from build123d import *

# Parameters (mm, degrees)
SKETCH_W        = 90
SKETCH_H        = 130
PAD_DEPTH       = 3
PAD007_DEPTH    = 3
PAD006_DEPTH    = 3
SKETCH014_R     = 5
SKETCH014_R_2   = 2
POCKET004_DEPTH = 10
SKETCH015_W     = 131.132767
SKETCH015_H     = 1
POCKET005_DEPTH = 100


with BuildPart() as pad007:
    # Sketch → Pad (new body)
    with BuildSketch(Plane.XY):
        with Locations((45, 65)):
            Rectangle(SKETCH_W, SKETCH_H)
    extrude(amount=PAD_DEPTH)

    # Sketch006 → Pad007 (new body)
    with BuildSketch(Plane.XY.offset(3)):
        with BuildLine():
            Line((0, 0), (90, 0))
            Line((90, 0), (90, 31.200001))
            Line((90, 87.7297593266), (90, 31.200001))
            Line((63.384261619, 87.7297593266), (90, 87.7297593266))
            ThreePointArc((73.2419105019, 65.6401585516), (70.414665309, 77.6228043326), (63.384261619, 87.7297593266))
            ThreePointArc((61.470024, 41.9983394519), (70.1525128312, 52.4267750542), (73.2419105019, 65.6401585516))
            Line((61.470024, 31.2), (61.470024, 41.9983394519))
            Line((0, 31.2), (61.470024, 31.2))
            Line((0, 31.2), (0, 0))
        make_face()
    extrude(amount=PAD007_DEPTH)


with BuildPart() as pocket005:
    # Sketch008 → Pad006 (new body)
    with BuildSketch(Plane(origin=(90, 130, 3), x_dir=(-1, 0, 0), z_dir=(0, 0, 1))):
        with BuildLine():
            Line((0, 0), (90, 0))
            Line((90, 0), (90, 31.200001))
            Line((90, 87.7297593266), (90, 31.200001))
            Line((63.384261619, 87.7297593266), (90, 87.7297593266))
            ThreePointArc((73.2419105019, 65.6401585516), (70.414665309, 77.6228043326), (63.384261619, 87.7297593266))
            ThreePointArc((61.470024, 41.9983394519), (70.1525128312, 52.4267750542), (73.2419105019, 65.6401585516))
            Line((61.470024, 31.2), (61.470024, 41.9983394519))
            Line((0, 31.2), (61.470024, 31.2))
            Line((0, 31.2), (0, 0))
        make_face()
    extrude(amount=PAD006_DEPTH)

    # Fusion: union Pad007
    add(pad007.part)

    # Sketch014 → Pocket004 (cut)
    with BuildSketch(Plane(origin=(0, 0, 0), x_dir=(1, 0, 0), z_dir=(0, 0, -1))):
        with Locations((45, -65)):
            Circle(SKETCH014_R)
        with Locations((7, -7)):
            Circle(SKETCH014_R_2)
        with Locations((7, -123)):
            Circle(SKETCH014_R_2)
        with Locations((83, -123)):
            Circle(SKETCH014_R_2)
        with Locations((83, -7)):
            Circle(SKETCH014_R_2)
    extrude(amount=-POCKET004_DEPTH, mode=Mode.SUBTRACT)

    # Sketch015 → Pocket005 (cut)
    with BuildSketch(Plane(origin=(0, 0, 0), x_dir=(0, -1, 0), z_dir=(-1, 0, 0))):
        with Locations((-65.5663835, 0.5)):
            Rectangle(SKETCH015_W, SKETCH015_H)
    extrude(amount=-POCKET005_DEPTH, mode=Mode.SUBTRACT)


solid = pocket005.part
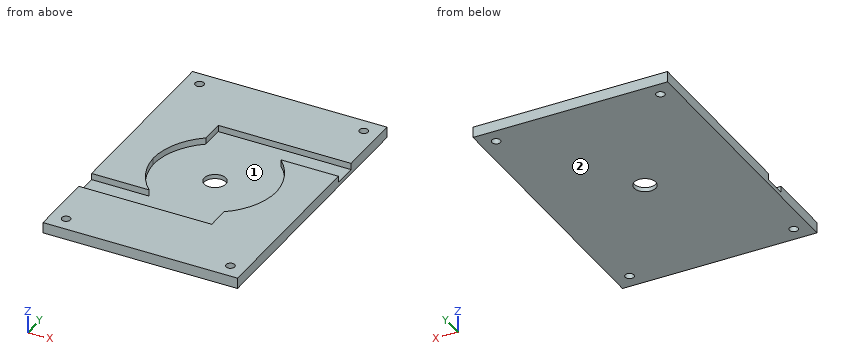
Work out the finished part from the listing and answer in its coordinate system (mm). Face numbers are marked on the shaded views. Coordinates: 2 decimals unless noted, no trailing zeros. Loops run counter-clockwise (first coordinate to the right, second up) from the corner with the lowest first, then second, coordinate; pieces in that order, holes last. Notation, with made-up numbers: (-33.75, -22) -> (-2.75, -22) arc R19 ccw to (-2.75, -6) -> close; hole circle Ø8 at (-17.75, 27.25). An arc over 180 degrees is marked (long way). Write each question's results on one line, items separated by ' | '. Start each with the question number.
1) The mould has two halves that part along Y. Classify the marked faces 1 and 2: pulls with the +Y half, pulls with the -Y half, needs draft (parallel to the pull), parting line crosses it, or undercut.
2) Consider line 1 along X through (y, z) = (123, 2); line 2 along Y through (x, z) = (83, 2.1); line 3 along Y through (x, z) = (42.5, 4). Determine where each line is inside the solid, lowest interval first.
3) Find section A-A on y = 123. Determine the outline of the cut face in (x, z), then the cut area to 3 significant figures.
4) Find section C-C on x = 45. Determine the outline of the cut face in (y, z), then the cut area to 3 significant figures.
5) Find section B-B on z = 4.9. Determine the outline of the cut face in (x, y), then the cut area to 3 significant figures.
6) Find section D-D on x = 7. Determine the outline of the cut face in (y, z).
7) A flat-ended cylindrical pin translates along its axis: P1, Ø2.5, axis at y = 36.5, z = 4.5, coming from the -X side. Find the tip coordinate at first contact, or state that the pin passes through.
Response values:
1) face 1: undercut | face 2: needs draft
2) line 1: x = 0 to 5, 9 to 81, 85 to 90 | line 2: y = 0 to 5, 9 to 121, 125 to 130 | line 3: y = 0 to 31.2, 98.8 to 130
3) outline: (0, 1) -> (5, 1) -> (5, 6) -> (0, 6) -> close; (9, 1) -> (81, 1) -> (81, 6) -> (9, 6) -> close; (85, 1) -> (90, 1) -> (90, 6) -> (85, 6) -> close | area: 410 mm^2
4) outline: (0, 1) -> (60, 1) -> (60, 3) -> (31.2, 3) -> (31.2, 6) -> (0, 6) -> close; (70, 1) -> (130, 1) -> (130, 6) -> (98.8, 6) -> (98.8, 3) -> (70, 3) -> close | area: 427 mm^2
5) outline: (0, 0) -> (90, 0) -> (90, 87.73) -> (63.38, 87.73) arc R32.93 cw to (73.24, 65.64) arc R29.47 cw to (61.47, 42) -> (61.47, 31.2) -> (0, 31.2) -> close; (0, 42.27) -> (26.62, 42.27) arc R32.93 cw to (16.76, 64.36) arc R29.47 cw to (28.53, 88) -> (28.53, 98.8) -> (90, 98.8) -> (90, 130) -> (0, 130) -> close; hole circle Ø4 at (7, 7); hole circle Ø4 at (7, 123); hole circle Ø4 at (83, 7); hole circle Ø4 at (83, 123) | area: 8,020 mm^2
6) outline: (0, 1) -> (5, 1) -> (5, 6) -> (0, 6) -> close; (9, 1) -> (121, 1) -> (121, 6) -> (42.27, 6) -> (42.27, 3) -> (31.2, 3) -> (31.2, 6) -> (9, 6) -> close; (125, 1) -> (130, 1) -> (130, 6) -> (125, 6) -> close
7) P1: stops at x = 61.47
